The model under review builds one solid part; all positions refer to its coordinate system, in mm. Face numbers are marked on the shaded views. A direction names the side the tool comes from. Round coordinates to 2 decimals unless told otherwise and drop trailing zeros. Write each loop counter-clockwise with the first axis right and the second up, starting at its lowest first coordinate (ties: lowest second). Pieces come first, ordered by that corner, then holes.
Item 1: To check wall thickness, follow L1, parallel to Y at x = 69.8, z = 0; L2, parallel to X at y = 7.5, z = 0; L3, parallel to X at y = 6, z = 2. State the ranges of each line that lie inside material, in increasing order.
Item 2: Add section D-D (z = 17.5). Give the boundary of the cut face in (x, y), plus the area to 3 significant figures.
Item 3: Machinability: for the marked faces 1 and 2, which of the approach directions +Z, -Z, +X, -X, +Y, -Y give a long, thin tool a straight path to every point of the face, cutting with its end or side? Answer none if there is none.
Item 4: Draft analysis for pull direction Z (two halves, no side actions). For the marked faces 3, 4, 5 and 6, state which applies: +Z half, -Z half, draft (parallel to the pull), parting line (faces both ways), or undercut.
Item 5: Add section B-B (z = -0.5). Give the boundary of the cut face in (x, y), plus the area to 3 significant figures.
Item 6: Clearance check with flat-ended pins moving along their axes: pin 1 Ø6 at (y, z) = (20, 6.5) entering from -X; pin 2 Ø1.5 at (x, y) = (17.5, 10.5) entering from +Z; pin 3 Ø16 at (x, z) = (0, 0) entering from +Y; pin 4 Ø3.5 at (y, z) = (-7.5, 0) entering from -X. State where each tip first meets the part, or that it passes through.
Item 7: Add section A-A (y = 2). Give the boundary of the cut face in (x, z), plus the area to 3 significant figures.
Item 8: Add section C-C (x = 21). Give the boundary of the cut face in (y, z).
```python
from build123d import *

# Parameters (mm, degrees)
SKETCH1_R           = 6.25
BOSS_EXTRUDE1_DEPTH = 10
SKETCH2_R           = 2.25
BOSS_EXTRUDE2_DEPTH = 5


with BuildPart() as part:
    # Sketch1 → Boss-Extrude1 (new body)
    with BuildSketch(Plane(origin=(0, 0, 0), x_dir=(1, 0, 0), z_dir=(0, 1, 0))):
        with BuildLine():
            Line((0, 11.25), (73.5, 30.944265644))
            Line((73.5, 30.944265644), (73.5, 20.59150384))
            Line((73.5, 20.59150384), (10.610062869, 3.740195973))
            ThreePointArc((10.610062869, 3.740195973), (11.25, 0), (10.610062869, -3.740195973))
            Line((10.610062869, -3.740195973), (73.5, -20.59150384))
            Line((73.5, -20.59150384), (73.5, -30.944265644))
            Line((73.5, -30.944265644), (0, -11.25))
            ThreePointArc((0, -11.25), (-11.25, 0), (0, 11.25))
        make_face()
        with Locations(Location((0, 0, 0), (0, 0, 270))):
            Circle(SKETCH1_R, mode=Mode.SUBTRACT)
    extrude(amount=BOSS_EXTRUDE1_DEPTH)

    # Sketch2 → Boss-Extrude2 (add)
    with BuildSketch(Plane(origin=(73.5, 0, 0), x_dir=(0, 0, -1), z_dir=(1, 0, 0))):
        with BuildLine():
            Line((-20.59150384, 10), (-6.25, 17.5))
            ThreePointArc((-6.25, 17.5), (0, 23.75), (6.25, 17.5))
            Line((6.25, 17.5), (20.59150384, 10))
            Line((20.59150384, 10), (20.59150384, 0))
            Line((20.59150384, 0), (6.25, -7.5))
            ThreePointArc((6.25, -7.5), (0, -13.75), (-6.25, -7.5))
            Line((-6.25, -7.5), (-20.59150384, 0))
            Line((-20.59150384, 0), (-20.59150384, 10))
        make_face()
        with Locations((0, 17.5)):
            Circle(SKETCH2_R, mode=Mode.SUBTRACT)
        with Locations((0, -7.5)):
            Circle(SKETCH2_R, mode=Mode.SUBTRACT)
    extrude(amount=-BOSS_EXTRUDE2_DEPTH)


solid = part.part
```
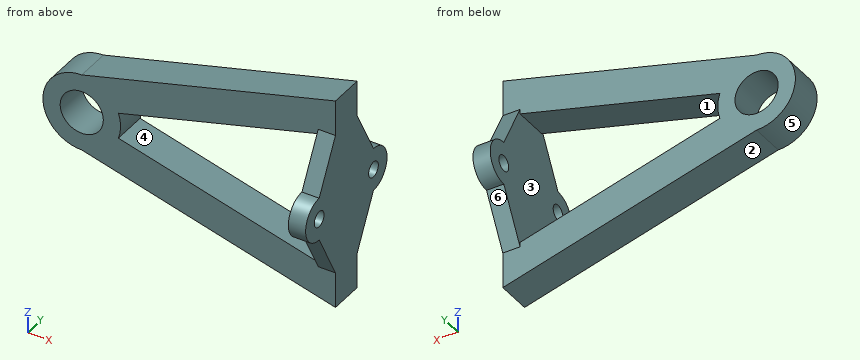
Numbers:
1. L1: y = -13.75 to -9.75, -5.25 to 15.25, 19.75 to 23.75
1. L2: x = -11.25 to -6.25, 6.25 to 11.25, 68.5 to 73.5
1. L3: x = -11.07 to -5.92, 5.92 to 11.07, 68.5 to 73.5
2. outline: (23.33, 0) - (61.96, 0) - (61.96, 10) - (23.33, 10) - close; (68.5, -1.62) - (73.5, -1.62) - (73.5, 11.62) - (68.5, 11.62) - close
2. area: 453 mm2
3. face 1: +Y, -Y
3. face 2: -Z, -X, +Y, -Y
4. face 3: undercut
4. face 4: undercut
4. face 5: parting line
4. face 6: -Z half
5. outline: (-11.24, 0) - (-6.23, 0) - (-6.23, 10) - (-11.24, 10) - close; (6.23, 0) - (11.24, 0) - (11.24, 10) - (6.23, 10) - close; (68.5, -13.73) - (73.5, -13.73) - (73.5, -9.69) - (68.5, -9.69) - close; (68.5, -5.31) - (73.5, -5.31) - (73.5, 15.31) - (68.5, 15.31) - close; (68.5, 19.69) - (73.5, 19.69) - (73.5, 23.73) - (68.5, 23.73) - close
5. area: 244 mm2
6. pin 1: stops at x = 68.5
6. pin 2: stops at z = 16.09
6. pin 3: stops at y = 10
6. pin 4: passes through
7. outline: (0, -11.25) - (73.5, -30.94) - (73.5, 30.94) - (0, 11.25) arc R11.25 ccw to start; hole circle Ø12.5 at (0, 0); hole (10.61, -3.74) - (68.5, -19.25) - (68.5, 19.25) - (10.61, 3.74) arc R11.25 cw to start
7. area: 1,850 mm2
8. outline: (0, -16.88) - (10, -16.88) - (10, -6.52) - (0, -6.52) - close; (0, 6.52) - (10, 6.52) - (10, 16.88) - (0, 16.88) - close
